The model under review builds one solid part; all positions refer to its coordinate system, in mm. Give positions to 0.01 mm unless a question says otherwise; leave off trailing zeros. Loops run counter-clockwise (first coordinate to the right, second up) from the corner with the lowest first, then second, coordinate; pieces in that order, holes last. Notation, with made-up numbers: (-25, -33) - (-10, -33) arc R20 ccw to (-10, -18) - close; hole circle Ø4 at (7.5, 7). An arc over 180 degrees is marked (long way). Return JSON: item names as keys, results as strings. Group by question number.
Autodesk Inventor part; units mm, degrees
ref_plane "YZ Plane" through (0, 0, 0) normal (1, 0, 0) x (0, 1, 0)
ref_plane "XZ Plane" through (0, 0, 0) normal (0, 1, 0) x (-1, 0, 0)
ref_plane "XY Plane" through (0, 0, 0) normal (0, 0, 1) x (1, 0, 0)
sketch "Sketch1" plane through (0, 0, 0) normal (0, 0, 1) x (1, 0, 0)
  line L0 (469.9, 22.205) -> (469.9, -34.945)
  line L1 (-99.06, -34.945) -> (-99.06, 22.205)
  circle A0 centre (-58.42, -4.7925) radius 13
  circle A1 centre (41.716, -4.7925) radius 13
  circle A2 centre (131.092, -4.7925) radius 13
  circle A3 centre (429.26, -4.7925) radius 13
  circle A4 centre (329.124, -4.7925) radius 13
  circle A5 centre (239.748, -4.7925) radius 13
  line L2 (-99.06, 28.36) -> (469.9, 28.36)
  line L3 (-99.06, -37.945) -> (469.9, -37.945)
  line L4 (-99.06, 22.205) -> (-99.06, 28.36)
  line L5 (-99.06, -37.945) -> (-99.06, -34.945)
  line L6 (469.9, -37.945) -> (469.9, -34.945)
  line L7 (469.9, 22.205) -> (469.9, 28.36)
  line L8 (-111.76, 41.06) -> (482.6, 41.06)
  line L9 (482.6, 41.06) -> (482.6, -50.645)
  line L10 (482.6, -50.645) -> (-111.76, -50.645)
  line L11 (-111.76, -50.645) -> (-111.76, 41.06)
  line L12 (508, 63.305) -> (508, -76.045)
  line L13 (508, -76.045) -> (-137.16, -76.045)
  line L14 (-137.16, -76.045) -> (-137.16, 63.305)
  line L15 (170, 41.06) -> (170, 66.46)
  line L16 (-137.16, 66.46) -> (508, 66.46)
  line L17 (508, 66.46) -> (508, 63.305)
  line L18 (-137.16, 66.46) -> (-137.16, 62)
  line L19 (-99.06, 4) -> (-111.76, 4)
  line L20 (-99.06, -10) -> (-111.76, -10)
  line L21 (176, 28.36) -> (176, 41.06)
  line L22 (191, 28.36) -> (191, 41.06)
  line L23 (176, -37.945) -> (176, -50.645)
  line L24 (191, -37.945) -> (191, -50.645)
  line L25 (469.9, 4) -> (482.6, 4)
  line L26 (469.9, -10) -> (482.6, -10)
  point P0 (0, 0)
  dimension "d4" = 26
  dimension "d6" = 26
  dimension "d8" = 26
  dimension "d10" = 26
  dimension "d12" = 26
  dimension "d14" = 26
  dimension "d16" = 568.96
  dimension "d18" = 40.64
  dimension "d19" = 140.776
  dimension "d20" = 230.152
  dimension "d21" = 230.152
  dimension "d22" = 40.64
  dimension "d23" = 140.776
  dimension "d29" = 66.305
  dimension "d45" = 33.1525
  dimension "d46" = 33.1525
  dimension "d47" = 33.1525
  dimension "d48" = 33.1525
  dimension "d49" = 33.1525
  dimension "d50" = 33.1525
  dimension "d52" = 12.7
  dimension "d53" = 12.7
  dimension "d54" = 25.4
  dimension "d56" = 25.4
  dimension "d57" = 15
extrude "Extrusion4" add sketch "Sketch1" along normal blind 9.525 contours L0 L6 L3 L5 L1 L4 L2 L7 | L25 L9 L26 L0 | L16 L17 L12 L13 L14 L18 | L2 L21 L8 L22 | L24 L10 L23 L3 | L1 L20 L11 L19
properties part number "side"
1) We need section B-B, the plane y = 16.5. Write out the cut boundary in (x, z) (3 decimals).
2) To check wall thickness, follow line 1 (Y direction, x = -57.5, z = 9.25) (3 decimals); line 2 (X direction, y = 39.5, z = 6.25); line 3 (Y direction, x = 263, z = 7.75) (3 decimals). State the ranges of each line that lie inside material, in increasing order.
3) We need section C-C, the plane z = 6.25. Count the separate pieces of the cut face and the enclosed holes in it, plus the area to 3 significant figures.
4) We need section D-D, the plane x = 329. Write out the cut boundary in (y, z) (3 decimals).
5) We need section A-A, the plane x = -58.42. Write out the cut boundary in (y, z) (1 decimal).
6) Draft analysis for pull direction X (two halves, no side actions). For faces 1 (the face through (416.273, -5.364, 4.696)), 2 (the face through (181, -4, 0)), state which applies: +X half, -X half, draft (parallel to the pull), parting line (faces both ways), or undercut.
Findings:
{
 "1": {"outline": "(-137.16, 0) - (-111.76, 0) - (-111.76, 9.525) - (-137.16, 9.525) - close; (-99.06, 0) - (469.9, 0) - (469.9, 9.525) - (-99.06, 9.525) - close; (482.6, 0) - (508, 0) - (508, 9.525) - (482.6, 9.525) - close"},
 "2": {"line 1": "y = -76.045 to -50.645, -37.945 to -17.76, 8.175 to 28.36, 41.06 to 66.46", "line 2": "x = -137.16 to -111.76, 176 to 191, 482.6 to 508", "line 3": "y = -76.045 to -50.645, -37.945 to 28.36, 41.06 to 66.46"},
 "3": {"separate pieces": "1", "enclosed holes": "10", "area": "72,700 mm^2"},
 "4": {"outline": "(-76.045, 0) - (-50.645, 0) - (-50.645, 9.525) - (-76.045, 9.525) - close; (-37.945, 0) - (-17.792, 0) - (-17.792, 9.525) - (-37.945, 9.525) - close; (8.207, 0) - (28.36, 0) - (28.36, 9.525) - (8.207, 9.525) - close; (41.06, 0) - (66.46, 0) - (66.46, 9.525) - (41.06, 9.525) - close"},
 "5": {"outline": "(-76, 0) - (-50.6, 0) - (-50.6, 9.5) - (-76, 9.5) - close; (-37.9, 0) - (-17.8, 0) - (-17.8, 9.5) - (-37.9, 9.5) - close; (8.2, 0) - (28.4, 0) - (28.4, 9.5) - (8.2, 9.5) - close; (41.1, 0) - (66.5, 0) - (66.5, 9.5) - (41.1, 9.5) - close"},
 "6": {"face 1": "undercut", "face 2": "draft"}
}
